Autodesk Inventor part; units mm, degrees
ref_plane "YZ Plane" through (0, 0, 0) normal (1, 0, 0) x (0, 1, 0)
ref_plane "XZ Plane" through (0, 0, 0) normal (0, 1, 0) x (-1, 0, 0)
ref_plane "XY Plane" through (0, 0, 0) normal (0, 0, 1) x (1, 0, 0)
sketch "Sketch1" plane through (0, 0, 0) normal (0, 1, 0) x (-1, 0, 0)
  circle A0 centre (0, 0) radius 11.25
  circle A1 centre (0, 0) radius 14.25
  circle A2 centre (0, 0) radius 30
  circle A3 centre (0, 0) radius 6.75
  dimension "d0" = 22.5
  dimension "d1" = 28.5
  dimension "d2" = 60
  dimension "d3" = 13.5
extrude "Extrusion1" add sketch "Sketch1" along normal blind 4.5 contours A0 | A1
sketch "Sketch2" plane through (0, 4.5, 0) normal (0, 1, 0) x (1, 0, 0)
  circle A0 centre (0, 0) radius 14.25
  circle A1 centre (0, 0) radius 11.25
  dimension "d6" = 22.5
extrude "Extrusion2" add sketch "Sketch2" along normal blind 8
sketch "Sketch3" plane through (0, 12.5, 0) normal (0, 1, 0) x (1, 0, 0)
  circle A0 centre (0, 0) radius 14.25
  circle A1 centre (0, 0) radius 25.25
  dimension "d9" = 50.5
extrude "Extrusion3" add sketch "Sketch3" against normal blind 3
chamfer "Chamfer2" distance 4.5 angle 45 1 edges at (6.75, 4.5, 0)
fillet "Fillet1" radius 5 1 edges at (14.25, 0, 0)
fillet "Fillet2" radius 2 1 edges at (-14.25, 9.5, 0)
fillet "Fillet3" radius 1 1 edges at (-25.25, 9.5, 0)
sketch "Sketch5" plane through (0, 9.5, 0) normal (0, -1, 0) x (1, 0, 0)
  circle A0 centre (0, 0) radius 16.25
  circle A1 centre (-20, 0) radius 1.5
  circle A2 centre (-20, 0) radius 3.75
  circle A3 centre (20, 0) radius 1.5
  circle A4 centre (0, -20) radius 1.5
  circle A5 centre (0, 20) radius 1.5
  dimension "d21" = 3
  dimension "d22" = 20
  dimension "d23" = 3
  dimension "d24" = 20
  dimension "d25" = 3
  dimension "d26" = 20
  dimension "d27" = 3
  dimension "d28" = 20
extrude "Extrusion4" cut sketch "Sketch5" against normal blind 11 contours A1 | A3 | A4 | A5
properties part number "supportoCuscinettoBasso"
Check sheet for the modelled part. Datum: model origin and axes. Units: mm. A direction names the side the tool comes from. Round coordinates to 2 decimals unless told otherwise and drop trailing zeros. Put each result on its own line as item: value. Start each with the question number.
1. Section check A-A (x = 0). Give the number of separate pieces and of enclosed holes in the cut face, plus the area to 3 significant figures.
2. Scan lines: probe 1 along Z at (x, y) = (0, 10.75); probe 2 along Z at (x, y) = (-2, 6.75); probe 3 along X at (y, z) = (7, 0). Record each from-to range of solid material in increasing order.
3. Access from +Z, -Z, +X, -X, +Y, -Y to the whole of each face (thin tool, end or side, straight path). Record for faces 1 (the face through (6, 0, -4)), 2 (the face through (-17, 9.5, 0)).
4. Gauge pin test, flat ends, axial feed: pin 1 (1.5 mm diameter, centred on x = 3, y = 8, fed in from +Z); pin 2 (11 mm diameter, centred on x = 3.5, z = -3.5, fed in from +Y); pin 3 (1.5 mm diameter, centred on y = 4, z = 5, fed in from -X). Record the tip position at first contact, or that the pin passes through.
5. Draft check along Z on faces 3 (the face through (5, 12.5, 11)), 4 (the face through (13.163, 6.232, -5.458)), 5 (the face through (5.19, 8.44, -9.98)). Enter one of: +Z half, -Z half, draft (parallel to the pull), parting line (faces both ways), or undercut.
Findings:
1. separate pieces: 4
1. enclosed holes: 0
1. area: 134 mm^2
2. probe 1: z = -25.25 to -21.5, -18.5 to -11.25, 11.25 to 18.5, 21.5 to 25.25
2. probe 2: z = -14.11 to -11.07, 11.07 to 14.11
2. probe 3: x = -14.25 to -11.25, 11.25 to 14.25
3. face 1: +Z, -Z, +X, -X, -Y
3. face 2: -Y
4. pin 1: stops at z = 14.4
4. pin 2: stops at y = 3.7
4. pin 3: stops at x = -13.53
5. face 3: draft
5. face 4: parting line
5. face 5: undercut
